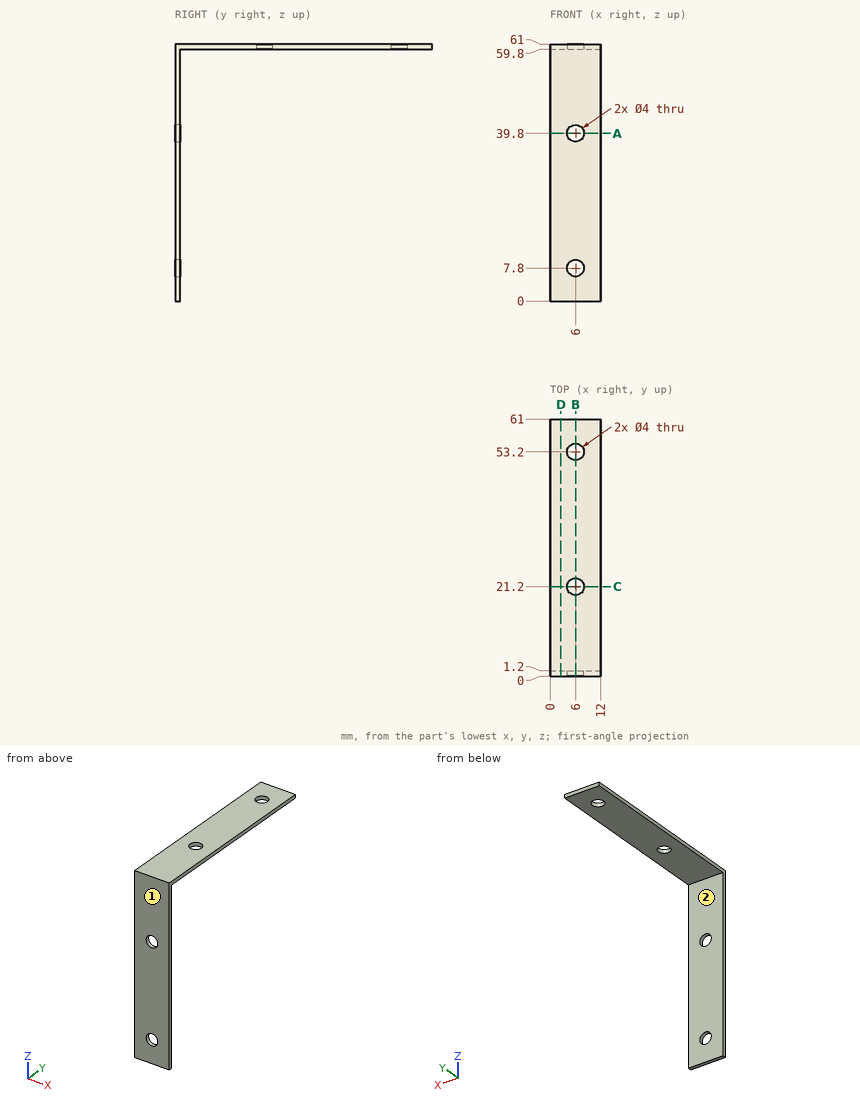
Drawing for the job (mm, zero at the part's lowest x, y, z). A direction names the side the tool comes from. Round coordinates to 2 decimals unless told otherwise and drop trailing zeros. Order: outer loops, then holes, each group sorted by start corner. A loop starts at its lowest first (then second) coordinate and runs counter-clockwise, first axis right, second up. Notation, with made-up numbers: M 15.25,60.5 L 27.25,60.5 A24 ccw 27.25,71.5 Z; hole C 20.5,30.5 d2. An arc over 180 degrees is marked long. Use one line per item in the form item = value.
Q1. Saw through at D-D on x = 2.5. Give the cut face in (y, z), then the cut area to 3 significant figures.
Recorded:
outline = M 0,0 L 1.2,0 L 1.2,59.8 L 61,59.8 L 61,61 L 0,61 Z
area = 145 mm^2
Q2. Which spindle directions (+Z, -Z, +X, -X, +Y, -Y) get a long thin tool onto all of the face, cutting with end or side? Do the marked faces 1 and 2. Say none if no direction does.
Recorded:
face_1 = +Z, -Z, +X, -X, -Y
face_2 = -Z, +X, -X, +Y
Q3. Flat gauge pins, fed straight in: P1, Ø6.5, axis at x = 6, z = 39.8, coming from the +Y side; P2, Ø3, axis at x = 4.5, y = 30, coming from the -Z side; P3, Ø1.5, axis at x = 5.5, z = 36, coming from the -Y side. Where does each tip first touch, or does it go through?
Recorded:
P1 = 1.2
P2 = 59.8
P3 = 0
Q4. Saw through at A-A on z = 39.8. Give the cut face in (x, y).
Recorded:
outline = M 0,0 L 4,0 L 4,1.2 L 0,1.2 Z; M 8,0 L 12,0 L 12,1.2 L 8,1.2 Z
Q5. Saw through at B-B on x = 6. Give the cut face in (y, z).
Recorded:
outline = M 0,0 L 1.2,0 L 1.2,5.8 L 0,5.8 Z; M 0,9.8 L 1.2,9.8 L 1.2,37.8 L 0,37.8 Z; M 0,41.8 L 1.2,41.8 L 1.2,59.8 L 19.2,59.8 L 19.2,61 L 0,61 Z; M 23.2,59.8 L 51.2,59.8 L 51.2,61 L 23.2,61 Z; M 55.2,59.8 L 61,59.8 L 61,61 L 55.2,61 Z
Q6. Saw through at C-C on y = 21.2. Give the cut face in (x, z), then the cut area to 3 significant figures.
Recorded:
outline = M 0,59.8 L 4,59.8 L 4,61 L 0,61 Z; M 8,59.8 L 12,59.8 L 12,61 L 8,61 Z
area = 9.60 mm^2
Q7. Probe L1, parallel to X at y = 0.35, z = 7.8; L2, parallel to Z at x = 9, y = 29; L3, parallel to Y at x = 6.5, z = 51.5. List the from-to ranges inside material, lowest first.
Recorded:
L1 = 0 to 4, 8 to 12
L2 = 59.8 to 61
L3 = 0 to 1.2
